Design review of the part built by this model. Coordinates are the model's own, in mm. Coordinates: 2 decimals unless noted, no trailing zeros. Write each loop counter-clockwise with the first axis right and the second up, starting at its lowest first coordinate (ties: lowest second). Pieces come first, ordered by that corner, then holes.
Q1. For L1, parallel to X at y = 5, z = 1.35 (3 decimals); L2, parallel to X at y = 48.5, z = 0.3; L3, parallel to X at y = -3, z = 0.25, list the stretches that pass through material, from the lowest coordinate up.
Q2. Take a section at B-B, the plane z = 1.4. State how many separate pieces and enclosed holes the cut face has, plus the area to 3 significant figures.
Q3. Take a section at A-A, the plane y = 5. Write out the cut boundary in (x, z) (3 decimals).
Q4. For pin 1 Ø1.8 at (x, y) = (-5, 47.5) entering from -Z, flat-tipped, find the tip position at first contact; note if it passes through.
Q5. Take a section at D-D, the plane x = -0.5. Write out the cut boundary in (y, z).
Q6. Take a section at C-C, the plane x = 5. Write out the cut boundary in (y, z), plus the area to 3 significant figures.
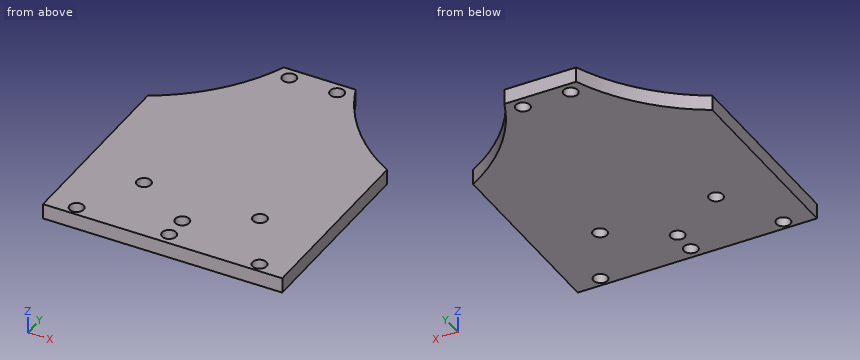
from build123d import *

# Parameters (mm, degrees)
SKETCH1_W           = 50
SKETCH1_H           = 30
SKETCH1_R           = 1.47
BOSS_EXTRUDE1_DEPTH = 3.18
BOSS_EXTRUDE2_DEPTH = 3.18
SKETCH3_R           = 1.47
CUT_EXTRUDE1_DEPTH  = 56.992074439
SKETCH4_R           = 1.47
CUT_EXTRUDE2_DEPTH  = 56.992074439


with BuildPart() as part:
    # Sketch1 → Boss-Extrude1 (new body)
    with BuildSketch(Plane.XY):
        with Locations((0, 5)):
            Rectangle(SKETCH1_W, SKETCH1_H)
        with Locations(Location((-12.125, 5, 0), (0, 0, 180))):
            Circle(SKETCH1_R, mode=Mode.SUBTRACT)
        with Locations(Location((12.125, 5, 0), (0, 0, 180))):
            Circle(SKETCH1_R, mode=Mode.SUBTRACT)
    extrude(amount=BOSS_EXTRUDE1_DEPTH)

    # Sketch2 → Boss-Extrude2 (add)
    with BuildSketch(Plane(origin=(0, 0, 0), x_dir=(-1, 0, 0), z_dir=(0, 0, -1))):
        with BuildLine():
            Line((-25, 20), (25, 20))
            Line((25, 20), (25, 30))
            ThreePointArc((25, 30), (14.540499974, 38.504187477), (7.5, 50))
            Line((7.5, 50), (-7.5, 50))
            ThreePointArc((-7.5, 50), (-14.540499974, 38.504187477), (-25, 30))
            Line((-25, 30), (-25, 20))
        make_face()
    extrude(amount=-BOSS_EXTRUDE2_DEPTH)

    # Sketch3 → Cut-Extrude1 (cut, through all)
    with BuildSketch(Plane(origin=(0, 0, 0), x_dir=(-1, 0, 0), z_dir=(0, 0, -1))):
        with Locations((-5, 47.5)):
            Circle(SKETCH3_R)
        with Locations((5, 47.5)):
            Circle(SKETCH3_R)
    extrude(amount=-CUT_EXTRUDE1_DEPTH, mode=Mode.SUBTRACT)

    # Sketch4 → Cut-Extrude2 (cut, through all)
    with BuildSketch(Plane(origin=(0, 0, 0), x_dir=(-1, 0, 0), z_dir=(0, 0, -1))):
        with Locations((0, -7.5)):
            Circle(SKETCH4_R)
        with Locations((-19.1461, -8)):
            Circle(SKETCH4_R)
        with Locations((0, -2.5)):
            Circle(SKETCH4_R)
        with Locations((19.0639, -8)):
            Circle(SKETCH4_R)
    extrude(amount=-CUT_EXTRUDE2_DEPTH, mode=Mode.SUBTRACT)


solid = part.part
Responses:
1. L1: x = -25 to -13.595, -10.655 to 10.655, 13.595 to 25
1. L2: x = -8.14 to -6.08, -3.92 to 3.92, 6.08 to 8.14
1. L3: x = -25 to -1.38, 1.38 to 25
2. separate pieces: 1
2. enclosed holes: 8
2. area: 2,510 mm2
3. outline: (-25, 0) - (-13.595, 0) - (-13.595, 3.18) - (-25, 3.18) - close; (-10.655, 0) - (10.655, 0) - (10.655, 3.18) - (-10.655, 3.18) - close; (13.595, 0) - (25, 0) - (25, 3.18) - (13.595, 3.18) - close
4. pin 1: passes through
5. outline: (-10, 0) - (-8.88, 0) - (-8.88, 3.18) - (-10, 3.18) - close; (-6.12, 0) - (-3.88, 0) - (-3.88, 3.18) - (-6.12, 3.18) - close; (-1.12, 0) - (50, 0) - (50, 3.18) - (-1.12, 3.18) - close
6. outline: (-10, 0) - (46.03, 0) - (46.03, 3.18) - (-10, 3.18) - close; (48.97, 0) - (50, 0) - (50, 3.18) - (48.97, 3.18) - close
6. area: 181 mm2
